Source: CAD feature listing. Evaluate the final solid. Frame: model axes, mm. A direction names the side the tool comes from. Coordinates: 2 decimals unless noted, no trailing zeros. Loops run counter-clockwise (first coordinate to the right, second up) from the corner with the lowest first, then second, coordinate; pieces in that order, holes last.
Autodesk Inventor part; units mm, degrees
ref_plane "YZ Plane" through (0, 0, 0) normal (1, 0, 0) x (0, 1, 0)
ref_plane "XZ Plane" through (0, 0, 0) normal (0, 1, 0) x (-1, 0, 0)
ref_plane "XY Plane" through (0, 0, 0) normal (0, 0, 1) x (1, 0, 0)
sketch "Sketch1" plane through (0, 0, 0) normal (0, 1, 0) x (-1, 0, 0)
  line L0 (0, -29.8704) -> (0, 29.8704)
  line L1 (-29.8704, 0) -> (29.8704, 0)
  line L2 (0, -21.336) -> (0, 21.336)
  line L3 (-21.336, 0) -> (21.336, 0)
  line L4 (15.24, -15.24) -> (4.191, -15.24)
  line L5 (-15.24, -15.24) -> (-4.191, -15.24)
  line L6 (15.24, 4.191) -> (12.827, 4.191)
  line L7 (12.827, -4.191) -> (15.24, -4.191)
  line L8 (-4.191, 12.827) -> (-4.191, 15.24)
  line L9 (4.191, 15.24) -> (4.191, 12.827)
  line L10 (-11.1208, -12.827) -> (-4.212, -5.9182)
  line L11 (-12.827, -11.1208) -> (-5.9182, -4.212)
  line L12 (-5.9182, 4.212) -> (-12.827, 11.1208)
  line L13 (-4.212, 5.9182) -> (-11.1208, 12.827)
  line L14 (-1.7062, 0) -> (0, 1.7062)
  line L15 (4.212, 5.9182) -> (11.1208, 12.827)
  line L16 (0, -1.7062) -> (1.7062, 0)
  line L17 (5.9182, 4.212) -> (12.827, 11.1208)
  line L18 (12.827, -11.1208) -> (5.9182, -4.212)
  line L19 (1.7062, 0) -> (0, 1.7062)
  line L20 (11.1208, -12.827) -> (4.212, -5.9182)
  line L21 (0, -1.7062) -> (-1.7062, 0)
  line L22 (4.191, -12.827) -> (4.191, -15.24)
  line L23 (-15.24, 4.191) -> (-12.827, 4.191)
  line L24 (-4.191, -15.24) -> (-4.191, -12.827)
  line L25 (-12.827, -4.191) -> (-15.24, -4.191)
  line L26 (11.1208, 12.827) -> (4.191, 12.827)
  line L27 (-4.191, 12.827) -> (-11.1208, 12.827)
  line L28 (-12.827, 11.1208) -> (-12.827, 4.191)
  line L29 (-12.827, -4.191) -> (-12.827, -11.1208)
  line L30 (-11.1208, -12.827) -> (-4.191, -12.827)
  line L31 (4.191, -12.827) -> (11.1208, -12.827)
  line L32 (12.827, -11.1208) -> (12.827, -4.191)
  line L33 (12.827, 4.191) -> (12.827, 11.1208)
  line L34 (-15.24, -15.24) -> (-15.24, -4.191)
  line L35 (-15.24, 4.191) -> (-15.24, 15.24)
  line L36 (15.24, -15.24) -> (4.191, -15.24)
  line L37 (-4.191, -15.24) -> (-15.24, -15.24)
  line L38 (15.24, 15.24) -> (15.24, 4.191)
  line L39 (15.24, -4.191) -> (15.24, -15.24)
  line L40 (-15.24, 15.24) -> (-4.191, 15.24)
  line L41 (4.191, 15.24) -> (15.24, 15.24)
  line L42 (4.212, 5.9182) -> (-4.212, 5.9182)
  line L43 (-5.9182, 4.212) -> (-5.9182, -4.212)
  line L44 (-4.212, -5.9182) -> (4.212, -5.9182)
  line L45 (5.9182, -4.212) -> (5.9182, 4.212)
  line L46 (5.9182, 5.9182) -> (-5.9182, -5.9182) construction
  line L47 (-5.9182, 5.9182) -> (5.9182, -5.9182) construction
  point P0 (0, 0)
  point P1 (0, 0)
  point P2 (0, -4.191)
  point P3 (-4.191, 0)
  point P4 (0, 4.191)
  point P5 (4.191, 0)
  dimension "d0" = 11.049
  dimension "d1" = 30.48
  dimension "d2" = 30.48
  dimension "d3" = 11.8364
  dimension "d4" = 11.8364
extrude "Extrusion1" add sketch "Sketch1" along normal blind 127 contours L44 L10 L30 L24 L5 L34 L25 L29 L11 L43 L1 L21 L0 | L0 L16 L1 L45 L18 L32 L7 L39 L4 L22 L31 L20 L44 | L19 L0 L42 L15 L26 L9 L41 L38 L6 L33 L17 L45 L1 | L1 L43 L12 L28 L23 L35 L40 L8 L27 L13 L42 L0 L14
properties part number "ProfileTwo"
Q1. Line query: line 1 along Z through (x, y) = (5.5, 84); line 2 along X through (y, z) = (115, 6.5); line 3 along Z through (x, y) = (0, 115.5). Output: solid intervals per line, ascending.
Q2. Contact query for flat-ended pins moving along their axis: pin 1 Ø2.5 at (x, y) = (-0.5, 39) entering from -Z; pin 2 Ø1 at (y, z) = (106.5, 1) entering from +X; pin 3 Ø2.5 at (y, z) = (44, 0) entering from -X; pin 4 Ø4 at (x, z) = (11, -2) entering from -Y. Output: stop coordinate, or through.
Q3. Section A-A, the plane x = -7.5. Return the cut outline in (y, z).
Q4. Section B-B, the plane z = -8. Return the cut outline in (x, y), plus the area to 3 significant figures.
Q5. Access query for faces 1 (the flat face through (-15.24, 63, -10)), 2 (the flat face through (7.618, 62.611, 9.324)), 3 (the flat face through (-5.918, 63, 0)). Directions: +Z, -Z, +X, -X, +Y, -Y. A direction counts if a zero-diameter tool reaches every point of the face in a straight line with its end or side. Return the directions, or none.
Q6. Draft query along X for faces 4 (the flat face through (-14, 63, -4.191)), 5 (the flat face through (-15.24, 63, 10)), 6 (the flat face through (-4.191, 63, 14)). Return one class per face: +X half, -X half, draft (parallel to the pull), parting line (faces both ways), or undercut.
Derived:
1. line 1: z = -15.24 to -12.83, -7.21 to 7.21, 12.83 to 15.24
1. line 2: x = -15.24 to -12.83, -8.21 to -4.79, 4.79 to 8.21, 12.83 to 15.24
1. line 3: z = -5.92 to -1.71, 1.71 to 5.92
2. pin 1: stops at z = -5.92
2. pin 2: stops at x = 5.92
2. pin 3: stops at x = -5.92
2. pin 4: passes through
3. outline: (0, -15.24) - (127, -15.24) - (127, -12.83) - (0, -12.83) - close; (0, -9.21) - (127, -9.21) - (127, -5.79) - (0, -5.79) - close; (0, 5.79) - (127, 5.79) - (127, 9.21) - (0, 9.21) - close; (0, 12.83) - (127, 12.83) - (127, 15.24) - (0, 15.24) - close
4. outline: (-15.24, 0) - (-12.83, 0) - (-12.83, 127) - (-15.24, 127) - close; (-9.71, 0) - (-6.29, 0) - (-6.29, 127) - (-9.71, 127) - close; (6.29, 0) - (9.71, 0) - (9.71, 127) - (6.29, 127) - close; (12.83, 0) - (15.24, 0) - (15.24, 127) - (12.83, 127) - close
4. area: 1,480 mm2
5. face 1: +Z, -Z, -X, +Y, -Y
5. face 2: +Y, -Y
5. face 3: -X, +Y, -Y
6. face 4: draft
6. face 5: -X half
6. face 6: undercut
